```python
from build123d import *

# Parameters (mm, degrees)
F0_W          = 88.9
F0_H          = 38.1
F1_DEPTH      = 44.45
F2_W          = 38.1
F2_H          = 33.02
F3_DEPTH      = 88.901
F4_W          = 5.5
F4_H          = 5.5
F5_DEPTH      = 36.068
F6_R          = 2.5
F7_DEPTH      = 37.3126
F7_DEPTH_BACK = 1
F9_DEPTH      = 38.1


with BuildPart() as f1:
    # F0 (on Front) → F1 (new body)
    with BuildSketch(Plane.XZ):
        with Locations((0.251959, 0.828608)):
            Rectangle(F0_W, F0_H)
    extrude(amount=F1_DEPTH)

    # F2 (on face) → F3 (cut, through all)
    with BuildSketch(Plane.YZ.offset(44.701959)):
        with Locations((-19.05, 3.368608)):
            Rectangle(F2_W, F2_H)
    extrude(amount=-F3_DEPTH, mode=Mode.SUBTRACT)

    # F4 (on face) → F5 (join)
    with BuildSketch(Plane.XY.offset(19.878608)):
        with Locations((41.951959, -41.7)):
            Rectangle(F4_W, F4_H)
    extrude(amount=-F5_DEPTH)

    # F6 (on face) → F7 (cut, two sides)
    with BuildSketch(Plane.XY.offset(19.878608)) as f7_sk:
        with Locations((41.951959, -41.7)):
            Circle(F6_R)
    extrude(amount=-F7_DEPTH, mode=Mode.SUBTRACT)
    extrude(f7_sk.sketch, amount=-F7_DEPTH_BACK, mode=Mode.SUBTRACT)

    # F8 (on face) → F9 (cut)
    with BuildSketch(Plane(origin=(0, 0, 0), x_dir=(-1, 0, 0), z_dir=(0, 1, 0))):
        Polygon((-34.6075, -14.208194), (-34.6075, -17.227376), (35.2425, -17.227376), (35.2425, -14.208194), (31.940609, -14.181392), (31.940609, -13.141392), (-31.302892, -13.141392), (-31.302892, -14.181392), align=None)
    extrude(amount=-F9_DEPTH, mode=Mode.SUBTRACT)


solid = f1.part
```
The model under review builds one solid part; all positions refer to its coordinate system, in mm. A direction names the side the tool comes from. Round coordinates to 2 decimals unless told otherwise and drop trailing zeros. Order: outer loops, then holes, each group sorted by start corner. A loop starts at its lowest first (then second) coordinate and runs counter-clockwise, first axis right, second up. Notation, with made-up numbers: (67.5, 48) -> (118.5, 48) arc R14 ccw to (118.5, 67) -> close; hole circle Ø3 at (2, 41.25). An arc over 180 degrees is marked (long way). Use a Markdown table: item, result.
Q1. We need section C-C on x = -20.5. Write out the cut boundary in (y, z).
Values:
| item | result |
|---|---|
| outline | (-44.45, -18.22) -> (0, -18.22) -> (0, -17.23) -> (-38.1, -17.23) -> (-38.1, 19.88) -> (-44.45, 19.88) -> close |
Q2. Clearance check with flat-ended pins moving along their axes: P1, Ø4, axis at x = 35, y = -18.5, coming from the +Z side; P2, Ø1.5, axis at x = 43, y = -42, coming from the +Z side; P3, Ø1, axis at x = 21, z = -8, coming from the +Y side. State where each tip first meets the part, or that it passes through.
Values:
| item | result |
|---|---|
| P1 | stops at z = -13.14 |
| P2 | stops at z = -17.43 |
| P3 | stops at y = -38.1 |
Q3. For line 1 (X direction, y = -35, z = -15.5); line 2 (Y direction, x = -40, z = -1); line 3 (Z direction, x = 8, y = -37), list the stretches that pass through material, from the lowest coordinate up.
Values:
| item | result |
|---|---|
| line 1 | x = -44.2 to -35.24, 34.61 to 44.7 |
| line 2 | y = -44.45 to -38.1 |
| line 3 | z = -18.22 to -17.23 |
Q4. We need section A-A on y = -41.7. Write out the cut boundary in (x, z).
Values:
| item | result |
|---|---|
| outline | (-44.2, -18.22) -> (44.7, -18.22) -> (44.7, 19.88) -> (44.45, 19.88) -> (44.45, -17.43) -> (39.45, -17.43) -> (39.45, 19.88) -> (-44.2, 19.88) -> close |
Q5. Tool access review of faces 1 (the flat face through (38, -19, -13.141)), 2 (the cylindrical face through (44.26, -42.66, 1.48)), 3 (the flat face through (0, -44.45, 1)): name each direction out of +Z, -Z, +X, -X, +Y, -Y from which nothing blocks a thin tool from reaching the whole face with its end or side.
Values:
| item | result |
|---|---|
| face 1 | +Z, +X, -X, +Y |
| face 2 | +Z |
| face 3 | +Z, -Z, +X, -X, -Y |
Q6. We need section D-D on y = -29.5. Write out the cut boundary in (x, z).
Values:
| item | result |
|---|---|
| outline | (-44.2, -18.22) -> (44.7, -18.22) -> (44.7, -13.14) -> (31.3, -13.14) -> (31.3, -14.18) -> (34.61, -14.21) -> (34.61, -17.23) -> (-35.24, -17.23) -> (-35.24, -14.21) -> (-31.94, -14.18) -> (-31.94, -13.14) -> (-44.2, -13.14) -> close |
Q7. We need section B-B on z = 16. Write out the cut boundary in (x, y), then the cut area to 3 significant figures.
Values:
| item | result |
|---|---|
| outline | (-44.2, -44.45) -> (44.7, -44.45) -> (44.7, -38.1) -> (-44.2, -38.1) -> close; hole circle Ø5 at (41.95, -41.7) |
| area | 545 mm^2 |
Q8. Mouldability with a two-part tool opening along Z and no side actions: class faces 4 (the flat face through (34.608, -19, -16)), 5 (the flat face through (-38, -19, -13.141)), 6 (the flat face through (0, -22, -18.221)), 7 (the flat face through (-35.242, -19, -16)) as +Z half, -Z half, draft (parallel to the pull), parting line (faces both ways), or undercut.
Values:
| item | result |
|---|---|
| face 4 | undercut |
| face 5 | +Z half |
| face 6 | -Z half |
| face 7 | undercut |
